Model file for the job. Use its own axes, mm. A direction names the side the tool comes from. Coordinates: 2 decimals unless noted, no trailing zeros. Write each loop counter-clockwise with the first axis right and the second up, starting at its lowest first coordinate (ties: lowest second). Pieces come first, ordered by that corner, then holes. Notation, with made-up numbers: (-11.5, 4.5) -> (38.5, 4.5) arc R29 ccw to (38.5, 38.5) -> close; hole circle Ø5 at (-14, 24.5). An arc over 180 degrees is marked (long way). Write item = value, one per line. Start each with the question number.
from build123d import *
from build123d.topology import SkipClean

# Parameters (mm, degrees)
BOSS_EXTRUDE3_OUTLINE_R = 3
BOSS_EXTRUDE3_DEPTH     = 97
SKETCH3_R               = 3
BOSS_EXTRUDE4_DEPTH     = 5
BOSS_EXTRUDE5_OUTLINE_R = 3
BOSS_EXTRUDE5_DEPTH     = 6
CUT_EXTRUDE2_DEPTH      = 6
CUT_EXTRUDE6_DEPTH      = 97
CUT_EXTRUDE9_DEPTH      = 97
SKETCH9_W               = 0.4
SKETCH9_H               = 1.8
SKETCH9_W_2             = 1.8
SKETCH9_H_2             = 0.4
BOSS_EXTRUDE6_DEPTH     = 97
SKETCH6_R               = 6.726787931
SKETCH6_R_2             = 3
SKETCH6_R_3             = 6.939010835
SKETCH6_R_4             = 7.483441293
SKETCH6_R_5             = 7.426515464
BOSS_EXTRUDE9_DEPTH     = 6
BOSS_EXTRUDE8_DEPTH     = 97


# Read off the part's stored shape, not the designer's step: Boss-Extrude3, Boss-Extrude5, Cut-Extrude2
with BuildPart() as part:
    # Boss-Extrude3 outline → Boss-Extrude3 (new body)
    with BuildSketch(Plane.XY):
        with BuildLine():
            ThreePointArc((-24.28, 72.228260397), (-55.793380191, 51.899313356), (-73.793224621, 19))
            Line((-73.793224621, 19), (-53.359615493, 19))
            add(Edge.make_bspline(
                [(-72.206415586, -24.344887517), (-69.541086329, -27.040667073), (-67.428574969, -29.089162938), (-64.355831171, -30.241441862), (-60.963009895, -31.073643307), (-59.042545022, -30.561519341), (-56.673971678, -29.217193929), (-54.241382838, -27.488775543), (-53, -25.105954954), (-53, -17.37432721), (-53.359615493, 19)],
                knots=[0, 0, 0, 0, 0, 0, 0, 0, 0, 0, 0, 1, 1, 1, 1, 1, 1, 1, 1, 1, 1, 1], degree=10))
            ThreePointArc((-72.206415586, -24.344887517), (-51.874242853, -55.816690411), (-19, -73.793224621))
            Line((-19, -73.793224621), (-19, -53))
            add(Edge.make_bspline(
                [(24.344887517, -72.206415586), (27.040667073, -69.541086329), (29.089162938, -67.428574969), (30.241441862, -64.355831171), (31.073643307, -60.963009895), (30.561519341, -59.042545022), (29.217193929, -56.673971678), (27.488775543, -54.241382838), (25.105954954, -53), (17.37432721, -53), (-19, -53)],
                knots=[0, 0, 0, 0, 0, 0, 0, 0, 0, 0, 0, 1, 1, 1, 1, 1, 1, 1, 1, 1, 1, 1], degree=10))
            ThreePointArc((24.344887517, -72.206415586), (55.816690411, -51.874242853), (73.793224621, -19))
            Line((73.793224621, -19), (53, -19))
            add(Edge.make_bspline(
                [(72.227927536, 24.280990174), (69.541086329, 27.040667073), (67.428574969, 29.089162938), (64.355831171, 30.241441862), (60.963009895, 31.073643307), (59.042545022, 30.561519341), (56.673971678, 29.217193929), (54.241382838, 27.488775543), (53, 25.105954954), (53, 17.37432721), (53, -19)],
                knots=[0, 0, 0, 0, 0, 0, 0, 0, 0, 0, 0, 1, 1, 1, 1, 1, 1, 1, 1, 1, 1, 1], degree=10))
            ThreePointArc((72.227927536, 24.280990174), (51.89893092, 55.793735933), (19, 73.793224621))
            Line((19, 73.793224621), (19, 53))
            add(Edge.make_bspline(
                [(-24.28, 72.228260397), (-27.040667073, 69.541086329), (-29.089162938, 67.428574969), (-30.241441862, 64.355831171), (-31.073643307, 60.963009895), (-30.561519341, 59.042545022), (-29.217193929, 56.673971678), (-27.488775543, 54.241382838), (-25.105954954, 53), (-17.37432721, 53), (19, 53)],
                knots=[0, 0, 0, 0, 0, 0, 0, 0, 0, 0, 0, 1, 1, 1, 1, 1, 1, 1, 1, 1, 1, 1], degree=10))
        make_face()
        with Locations((-30, -59)):
            Circle(BOSS_EXTRUDE3_OUTLINE_R, mode=Mode.SUBTRACT)
        Polygon((-38.9, -51.6), (-51.6, -51.6), (-51.6, -38.9), (-50, -38.9), (-50, 38.9), (-51.6, 38.9), (-51.6, 51.6), (-38.9, 51.6), (-38.9, 50), (38.9, 50), (38.9, 51.6), (51.6, 51.6), (51.6, 38.9), (50, 38.9), (50, -38.9), (51.6, -38.9), (51.6, -51.6), (38.9, -51.6), (38.9, -50), (-38.9, -50), align=None, mode=Mode.SUBTRACT)
        with Locations((59, -30)):
            Circle(BOSS_EXTRUDE3_OUTLINE_R, mode=Mode.SUBTRACT)
        with Locations((-59.359615493, 30)):
            Circle(BOSS_EXTRUDE3_OUTLINE_R, mode=Mode.SUBTRACT)
        with Locations((30, 59)):
            Circle(BOSS_EXTRUDE3_OUTLINE_R, mode=Mode.SUBTRACT)
    extrude(amount=BOSS_EXTRUDE3_DEPTH)

    # Sketch3 → Boss-Extrude4 (add)
    with BuildSketch(Plane.XY.offset(97)):
        with Locations(Location((-59.359615493, 30, 0), (0, 0, 180))):
            Circle(SKETCH3_R)
    extrude(amount=BOSS_EXTRUDE4_DEPTH)


with BuildPart() as boss_extrude4_kept_piece:
    # of the separate pieces the step leaves, the one the design keeps (boss_extrude4_pieces_kept)
    add(part.part.solids().sort_by_distance((-24.28, 72.228260397, 0))[0])

    # Boss-Extrude5 outline → Boss-Extrude5 (add)
    with BuildSketch(Plane.XY):
        with Locations((-59.359615493, 30)):
            Circle(BOSS_EXTRUDE5_OUTLINE_R)
    extrude(amount=BOSS_EXTRUDE5_DEPTH)

    # Cut-Extrude2 outline → Cut-Extrude2 (cut)
    with BuildSketch(Plane.XY):
        Polygon((-32.75, -54.236860279), (-35.5, -59), (-32.75, -63.763139721), (-27.25, -63.763139721), (-24.5, -59), (-27.25, -54.236860279), align=None)
        Polygon((59, -24.5), (54.236860279, -27.25), (54.236860279, -32.75), (59, -35.5), (63.763139721, -32.75), (63.763139721, -27.25), align=None)
        Polygon((-59.359615493, 35.5), (-64.122755214, 32.75), (-64.122755214, 27.25), (-59.359615493, 24.5), (-54.596475772, 27.25), (-54.596475772, 32.75), align=None)
        Polygon((32.75, 63.763139721), (27.25, 63.763139721), (24.5, 59), (27.25, 54.236860279), (32.75, 54.236860279), (35.5, 59), align=None)
    extrude(amount=CUT_EXTRUDE2_DEPTH, mode=Mode.SUBTRACT)

    # Sketch7 → Cut-Extrude6 (cut)
    with BuildSketch(Plane.XY.offset(97)):
        Polygon((-38.7, -51.8), (-51.8, -51.8), (-51.8, -38.7), (-50.2, -38.7), (-50.2, 38.7), (-51.8, 38.7), (-51.8, 51.8), (-38.7, 51.8), (-38.7, 50.2), (38.7, 50.2), (38.7, 51.8), (51.8, 51.8), (51.8, 38.7), (50.2, 38.7), (50.2, -38.7), (51.8, -38.7), (51.8, -51.8), (38.7, -51.8), (38.7, -50.2), (-38.7, -50.2), align=None)
        Polygon((-38.9, -51.6), (-51.6, -51.6), (-51.6, -38.9), (-50, -38.9), (-50, 38.9), (-51.6, 38.9), (-51.6, 51.6), (-38.9, 51.6), (-38.9, 50), (38.9, 50), (38.9, 51.6), (51.6, 51.6), (51.6, 38.9), (50, 38.9), (50, -38.9), (51.6, -38.9), (51.6, -51.6), (38.9, -51.6), (38.9, -50), (-38.9, -50), align=None, mode=Mode.SUBTRACT)
    extrude(amount=-CUT_EXTRUDE6_DEPTH, mode=Mode.SUBTRACT)

    # Sketch8 → Cut-Extrude9 (cut)
    with BuildSketch(Plane.XY.offset(97)):
        Polygon((-51.8, 38.7), (-51.8, 51.8), (-38.7, 51.8), (-38.7, 52), (-52, 52), (-52, 38.7), align=None)
        Polygon((-51.8, -38.7), (-51.8, -51.8), (-38.7, -51.8), (-38.7, -52), (-52, -52), (-52, -38.7), align=None)
        Polygon((51.8, -38.7), (51.8, -51.8), (38.7, -51.8), (38.7, -52), (52, -52), (52, -38.7), align=None)
        Polygon((51.8, 38.7), (51.8, 51.8), (38.7, 51.8), (38.7, 52), (52, 52), (52, 38.7), align=None)
    extrude(amount=-CUT_EXTRUDE9_DEPTH, mode=Mode.SUBTRACT)

    # Sketch9 → Boss-Extrude6 (add)
    with BuildSketch(Plane.XY.offset(97)):
        with Locations((-38.9, 51.1)):
            Rectangle(SKETCH9_W, SKETCH9_H)
        with Locations((-51.1, 38.9)):
            Rectangle(SKETCH9_W_2, SKETCH9_H_2)
        with Locations((38.9, 51.1)):
            Rectangle(SKETCH9_W, SKETCH9_H)
        with Locations((51.1, 38.9)):
            Rectangle(SKETCH9_W_2, SKETCH9_H_2)
        with Locations((51.1, -38.9)):
            Rectangle(SKETCH9_W_2, SKETCH9_H_2)
        with Locations((38.9, -51.1)):
            Rectangle(SKETCH9_W, SKETCH9_H)
        with Locations((-51.1, -38.9)):
            Rectangle(SKETCH9_W_2, SKETCH9_H_2)
        with Locations((-38.9, -51.1)):
            Rectangle(SKETCH9_W, SKETCH9_H)
    extrude(amount=-BOSS_EXTRUDE6_DEPTH)

    # Sketch6 → Boss-Extrude9 (add)
    # profile 1 of 4: a face of its own
    with SkipClean():  # the faces are left unmerged after this step: merging them gives an invalid solid
        with BuildSketch(Plane(origin=(0, 0, 0), x_dir=(-1, 0, 0), z_dir=(0, 0, -1))):
            with Locations((-30, 59)):
                Circle(SKETCH6_R)
            with Locations((-30, 59)):
                Circle(SKETCH6_R_2, mode=Mode.SUBTRACT)
        # profile 2 of 4: a face of its own
        with BuildSketch(Plane(origin=(0, 0, 0), x_dir=(-1, 0, 0), z_dir=(0, 0, -1))):
            with Locations((59.359615493, 30)):
                Circle(SKETCH6_R_3)
            with Locations((59.359615493, 30)):
                Circle(SKETCH6_R_2, mode=Mode.SUBTRACT)
        # profile 3 of 4: a face of its own
        with BuildSketch(Plane(origin=(0, 0, 0), x_dir=(-1, 0, 0), z_dir=(0, 0, -1))):
            with Locations((30, -59)):
                Circle(SKETCH6_R_4)
            with Locations((30, -59)):
                Circle(SKETCH6_R_2, mode=Mode.SUBTRACT)
        # profile 4 of 4: a face of its own
        with BuildSketch(Plane(origin=(0, 0, 0), x_dir=(-1, 0, 0), z_dir=(0, 0, -1))):
            with Locations((-59, -30)):
                Circle(SKETCH6_R_5)
            with Locations((-59, -30)):
                Circle(SKETCH6_R_2, mode=Mode.SUBTRACT)
        extrude(amount=-BOSS_EXTRUDE9_DEPTH)

    # Sketch11 → Boss-Extrude8 (add)
    with SkipClean():  # the faces are left unmerged after this step: merging them gives an invalid solid
        with BuildSketch(Plane.XY.offset(97)):
            with BuildLine():
                ThreePointArc((-73.793224621, 19), (-76.148989183, -2.787731402), (-72.206415586, -24.344887517))
                add(Edge.make_bspline(
                    [(-53.359615493, 19), (-53, -17.37432721), (-53, -25.105954954), (-54.241382838, -27.488775543), (-56.673971678, -29.217193929), (-59.042545022, -30.561519341), (-60.963009895, -31.073643307), (-64.355831171, -30.241441862), (-67.428574969, -29.089162938), (-69.541086329, -27.040667073), (-72.206415586, -24.344887517)],
                    knots=[0, 0, 0, 0, 0, 0, 0, 0, 0, 0, 0, 1, 1, 1, 1, 1, 1, 1, 1, 1, 1, 1], degree=10))
                Line((-53.359615493, 19), (-73.793224621, 19))
            make_face()
        extrude(amount=BOSS_EXTRUDE8_DEPTH)


with BuildPart() as boss_extrude8_kept_piece:
    # of the separate pieces the step leaves, the one the design keeps (boss_extrude8_pieces_kept)
    add(boss_extrude4_kept_piece.part.solids().sort_by_distance((-24.28, 72.228260397, 0))[0])


solid = boss_extrude8_kept_piece.part
(1) Saw through at B-B (z = 8). State how many separate pieces and enclosed holes the cut face has, then the cut area to 3 significant figures.
(2) Mould opens along Y. For faces 1 (the face through (-19, -64, 48)), 2 (the face through (52.29, 55.43, 47.82)), 3 (the face through (45, -52, 49)) say: released by +Y, released by -Y, zero draft, split by the parting line, or undercut.
(3) Drill centre lines: line 1 along Y through (x, z) = (0, 57.5); line 2 along X through (y, z) = (-30, 45); line 3 along X through (y, z) = (-59, 63). Where is each one in solid material? Low to high.
(4) Saw through at A-A (y = -46.5). Give the cut face in (x, z), then the cut area to 3 significant figures.
(5) 3-axis set-ups, long thin cutter, end or side, ignore diameter. For faces 4 (the face through (-64, 19, 48)), 5 (the face through (-50.2, -1, 49)), 6 (the face through (19, 64, 48)): which of +Z, -Z, +X, -X, +Y, -Y reach the whole face in a straight line?
(6) Drop flat-ended pins along their axis: pin 1 Ø12 at (y, z) = (-28, 13) entering from -X; pin 2 Ø10 at (y, z) = (19.5, 73) entering from +X; pin 3 Ø5 at (x, z) = (-20, 73.5) entering from +Y. Give the stop position or say it passes through.
Returned:
q1.separate_pieces = 1
q1.enclosed_holes = 5
q1.area = 3,820 mm2
q2.face_1 = zero draft
q2.face_2 = released by +Y
q2.face_3 = undercut
q3.line_1 = -53.04 to -50.2, 50.2 to 53.04
q3.line_2 = -70.05 to -50.2, 50.2 to 56, 62 to 70.05
q3.line_3 = -48.22 to -33, -27 to -19, 29.41 to 48.22
q4.outline = (-60.37, 0) -> (-52, 0) -> (-52, 97) -> (-60.37, 97) -> close; (52, 0) -> (60.37, 0) -> (60.37, 97) -> (52, 97) -> close
q4.area = 1,620 mm2
q5.face_4 = +Z, -Z, -X
q5.face_5 = +Z, -Z
q5.face_6 = +Z, -Z, +Y
q6.pin_1 = -72.21
q6.pin_2 = 72.23
q6.pin_3 = 54.3
